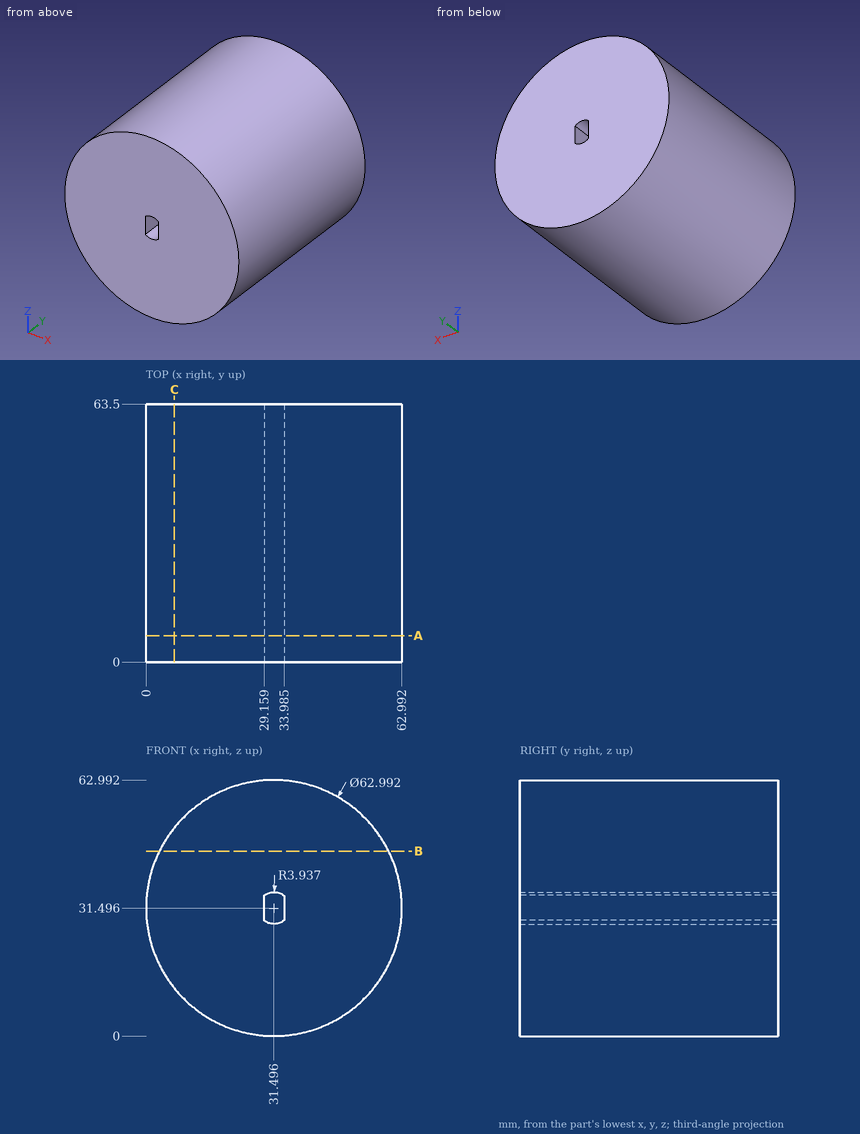
Here's the drawing with two shaded views (mm, measured from the low corner). I have some questions. Round coordinates to 2 decimals unless told otherwise and drop trailing zeros. Loops run counter-clockwise (first coordinate to the right, second up) from the corner with the lowest first, then second, coordinate; pieces in that order, holes last.
Item 1: Suppose I cut it at A-A, the plane y = 6.5. Write out the boundary of the cut face in (x, z) (1 decimal).
Item 2: Will these pins go through, and if not, where does the flat tip stop? pin 1 Ø1.5 at (x, y) = (21, 13.5) entering from +Z; pin 2 Ø8 at (x, y) = (38.5, 29) entering from -Z; pin 3 Ø5 at (y, z) = (52, 55) entering from -X.
Item 3: Suppose I cut it at C-C, the plane x = 7. Write out the boundary of the cut face in (y, z), then the cut area to 3 significant figures.
Item 4: Suppose I cut it at B-B, the plane z = 45.5. Write out the boundary of the cut face in (x, y), then the cut area to 3 significant figures.
Item 5: Please list where these lines run through material, in increasing order: L1, parallel to X at y = 18, z = 31 (1 decimal); L2, parallel to X at y = 58, z = 35 (1 decimal); L3, parallel to X at y = 47, z = 12.
Reported:
1. outline: circle Ø63 at (31.5, 31.5); hole (29.2, 28.3) arc R3.9 ccw to (34, 28.4) - (34, 34.5) arc R3.9 ccw to (29.2, 34.7) - close
2. pin 1: stops at z = 61.45
2. pin 2: stops at z = 0.14
2. pin 3: stops at x = 8.03
3. outline: (0, 11.7) - (63.5, 11.7) - (63.5, 51.29) - (0, 51.29) - close
3. area: 2,510 mm2
4. outline: (3.28, 0) - (59.71, 0) - (59.71, 63.5) - (3.28, 63.5) - close
4. area: 3,580 mm2
5. L1: x = 0 to 29.2, 34 to 63
5. L2: x = 0.2 to 29.7, 33.3 to 62.8
5. L3: x = 6.76 to 56.23
